from build123d import *

# Parameters (mm, degrees)
ESBO_O1_W                = 240
ESBO_O1_H                = 50
ESBO_O1_R                = 11
RESSALTO_EXTRUS_O1_DEPTH = 10
FILETE1_R                = 5


with BuildPart() as part:
    # Esboço1 → Ressalto-extrusão1 (new body)
    with BuildSketch(Plane.XY):
        with Locations((120, 25)):
            Rectangle(ESBO_O1_W, ESBO_O1_H)
        with Locations((20, 25)):
            Circle(ESBO_O1_R, mode=Mode.SUBTRACT)
        with Locations((220, 25)):
            Circle(ESBO_O1_R, mode=Mode.SUBTRACT)
    extrude(amount=RESSALTO_EXTRUS_O1_DEPTH)

    # Filete1
    filete1_edges = [part.edges().sort_by_distance(p)[0] for p in [
        (120, 50, 10),
        (0, 25, 10),
        (120, 0, 10),
        (0, 25, 0),
        (120, 50, 0),
        (240, 25, 0),
        (120, 0, 0),
        (0, 0, 5),
        (0, 50, 5),
        (240, 50, 5),
        (240, 0, 5),
        (240, 25, 10),
    ]]
    fillet(filete1_edges, radius=FILETE1_R - 0.0001)  # a hair under: the kernel refuses the full size


solid = part.part
Verification items for the finished model (mm, model axes). Round coordinates to 2 decimals unless told otherwise and drop trailing zeros. Order: outer loops, then holes, each group sorted by start corner. A loop starts at its lowest first (then second) coordinate and runs counter-clockwise, first axis right, second up. Notation, with made-up numbers: (53.25, -39.75) -> (73.25, -39.75) arc R28 ccw to (73.25, -8.75) -> close; hole circle Ø9 at (83, -22). An arc over 180 degrees is marked (long way). Put each result on its own line as item: value.
1) Section check B-B (y = 25). Give the number of separate pieces and of enclosed holes in the cut face, then the cut area to 3 significant figures.
Final values:
separate pieces: 3
enclosed holes: 0
area: 1,940 mm^2
2) Section check C-C (z = 8.25). Record the cut outline in (x, y).
Final values:
outline: (1.2, 5) arc R3.8 ccw to (5, 1.2) -> (235, 1.2) arc R3.8 ccw to (238.8, 5) -> (238.8, 45) arc R3.8 ccw to (235, 48.8) -> (5, 48.8) arc R3.8 ccw to (1.2, 45) -> close; hole circle Ø22 at (20, 25); hole circle Ø22 at (220, 25)
3) Mould release check, pull along Y, two halves, no side actions. Record for faces 1 (the cylindrical face through (122, 1, 8)), 2 (the cylindrical face through (1, 25, 2)), 3 (the cylindrical face through (25.076, 15.241, 4.93)): +Y half, -Y half, draft (parallel to the pull), parting line (faces both ways), or undercut.
Final values:
face 1: -Y half
face 2: draft
face 3: undercut
4) Material ranges on line 1 (X direction, y = 28, z = 7.25); line 2 (Y direction, x = 20, z = 5); line 3 (X direction, y = 30, z = 4.75), recorded low to high.
Final values:
line 1: x = 0.53 to 9.42, 30.58 to 209.42, 230.58 to 239.47
line 2: y = 0 to 14, 36 to 50
line 3: x = 0.01 to 10.2, 29.8 to 210.2, 229.8 to 239.99
5) Depth check by flat-ended pin: pin 1 (20 mm diameter, centred on x = 20, y = 25, fed in from -Z); pin 2 (4 mm diameter, centred on y = 11, z = 2.5, fed in from -X); pin 3 (1.5 mm diameter, centred on y = 27, z = 2.5, fed in from -X); pin 4 (1.5 mm diameter, centred on y = 7, z = 8, fed in from +X). Enter the tip coordinate at first touch or a pass-through.
Final values:
pin 1: passes through
pin 2: stops at x = 0.03
pin 3: stops at x = 0.32
pin 4: stops at x = 239.47
